Verification items for the finished model (mm, model axes). A direction names the side the tool comes from. Give positions to 0.01 mm unless a question says otherwise; leave off trailing zeros. Write each loop counter-clockwise with the first axis right and the second up, starting at its lowest first coordinate (ties: lowest second). Pieces come first, ordered by that corner, then holes. Notation, with made-up numbers: (-13.5, -5.75) - (35.5, -5.75) arc R13 cw to (35.5, -0.75) - close; hole circle Ø11 at (-3.5, 13). An arc over 180 degrees is marked (long way). Answer as a JSON object with one key per item and string values. Group by question number.
Item 1: Go/stop test with flat-tipped pins: pin 1 (7 mm diameter, centred on y = 0, z = 12.7, fed in from +X) (3 decimals); pin 2 (2 mm diameter, centred on x = -1.5, y = -6, fed in from +Z) (3 decimals); pin 3 (3 mm diameter, centred on x = 1.524, y = 0, fed in from -Z). Record where each tip stops, or that it passes through.
Item 2: Sectioned sample at B-B, the plane y = 12.7. Record the boundary of the cut face in (x, z) (3 decimals).
Item 3: Tool access check on faces 1 (the face through (-6.35, -0.3, 9.7)), 2 (the face through (-3.175, 0, 17)). Record the directions out of +Z, -Z, +X, -X, +Y, -Y that give a thin tool (end or side, any length) a straight path to the whole face; none if there is none.
Item 4: Sectioned sample at D-D, the plane x = 3.75. Record the boundary of the cut face in (y, z) (3 decimals).
Item 5: Scan lines: line 1 along X through (y, z) = (-12.7, 0.7); line 2 along Z through (x, y) = (-5.25, -12.7); line 3 along Y through (x, z) = (-3.25, 12.25). Record each from-to range of solid material in increasing order. Write a range as [from, to].
Item 6: Draft check along Y on faces 3 (the face through (-4, 19.05, 9)), 4 (the face through (5, 0, 3.175)), 5 (the face through (-4.74, 15.244, 13.501)). Enter one of: +Y half, -Y half, draft (parallel to the pull), parting line (faces both ways), or undercut.
Item 7: Sectioned sample at A-A, the plane z = 12.7. Record the boundary of the cut face in (x, y) (3 decimals), and give its area (3 significant figures).
Item 8: Sectioned sample at C-C, the plane z = 2.5. Record the boundary of the cut face in (x, y).
```python
from build123d import *

# Parameters (mm, degrees)
SKETCH1_W           = 19.05
SKETCH1_H           = 38.1
SKETCH1_R           = 2.667
BOSS_EXTRUDE1_DEPTH = 3.175
SKETCH2_W           = 3.175
SKETCH2_H           = 38.1
BOSS_EXTRUDE2_DEPTH = 22.225
SKETCH4_R           = 2.667
CUT_EXTRUDE1_DEPTH  = 36.497579143


with BuildPart() as part:
    # Sketch1 → Boss-Extrude1 (new body)
    with BuildSketch(Plane.XY):
        with Locations((3.175, 0)):
            Rectangle(SKETCH1_W, SKETCH1_H)
        with Locations(Location((1.524, -12.7, 0), (0, 0, 180))):
            Circle(SKETCH1_R, mode=Mode.SUBTRACT)
        with Locations(Location((1.524, 0, 0), (0, 0, 180))):
            Circle(SKETCH1_R, mode=Mode.SUBTRACT)
        with Locations(Location((1.524, 12.7, 0), (0, 0, 180))):
            Circle(SKETCH1_R, mode=Mode.SUBTRACT)
    extrude(amount=BOSS_EXTRUDE1_DEPTH)

    # Sketch2 → Boss-Extrude2 (add)
    with BuildSketch(Plane.XY.offset(3.175)):
        with Locations((-4.7625, 0)):
            Rectangle(SKETCH2_W, SKETCH2_H)
    extrude(amount=BOSS_EXTRUDE2_DEPTH)

    # Sketch4 → Cut-Extrude1 (cut, through all)
    with BuildSketch(Plane(origin=(-3.175, 0, 0), x_dir=(0, 0, -1), z_dir=(1, 0, 0))):
        with Locations(Location((-12.7, 0, 0), (0, 0, 90))):
            Circle(SKETCH4_R)
        with Locations(Location((-12.7, 12.7, 0), (0, 0, 90))):
            Circle(SKETCH4_R)
        with Locations(Location((-12.7, -12.7, 0), (0, 0, 90))):
            Circle(SKETCH4_R)
    extrude(amount=-CUT_EXTRUDE1_DEPTH, mode=Mode.SUBTRACT)


solid = part.part
```
Geometry check:
{
 "1": {"pin 1": "x = -3.175", "pin 2": "z = 3.175", "pin 3": "through"},
 "2": {"outline": "(-6.35, 0) - (-1.143, 0) - (-1.143, 3.175) - (-3.175, 3.175) - (-3.175, 10.033) - (-6.35, 10.033) - close; (-6.35, 15.367) - (-3.175, 15.367) - (-3.175, 25.4) - (-6.35, 25.4) - close; (4.191, 0) - (12.7, 0) - (12.7, 3.175) - (4.191, 3.175) - close"},
 "3": {"face 1": "+Z, -Z, -X, +Y, -Y", "face 2": "+Z, +X, +Y, -Y"},
 "4": {"outline": "(-19.05, 0) - (-14.169, 0) - (-14.169, 3.175) - (-19.05, 3.175) - close; (-11.231, 0) - (-1.469, 0) - (-1.469, 3.175) - (-11.231, 3.175) - close; (1.469, 0) - (11.231, 0) - (11.231, 3.175) - (1.469, 3.175) - close; (14.169, 0) - (19.05, 0) - (19.05, 3.175) - (14.169, 3.175) - close"},
 "5": {"line 1": "[-6.35, -1.14], [4.19, 12.7]", "line 2": "[0, 10.03], [15.37, 25.4]", "line 3": "[-19.05, -15.33], [-10.07, -2.63], [2.63, 10.07], [15.33, 19.05]"},
 "6": {"face 3": "+Y half", "face 4": "draft", "face 5": "undercut"},
 "7": {"outline": "(-6.35, -19.05) - (-3.175, -19.05) - (-3.175, -15.367) - (-6.35, -15.367) - close; (-6.35, -10.033) - (-3.175, -10.033) - (-3.175, -2.667) - (-6.35, -2.667) - close; (-6.35, 2.667) - (-3.175, 2.667) - (-3.175, 10.033) - (-6.35, 10.033) - close; (-6.35, 15.367) - (-3.175, 15.367) - (-3.175, 19.05) - (-6.35, 19.05) - close", "area": "70.2 mm^2"},
 "8": {"outline": "(-6.35, -19.05) - (12.7, -19.05) - (12.7, 19.05) - (-6.35, 19.05) - close; hole circle Ø5.33 at (1.52, -12.7); hole circle Ø5.33 at (1.52, 0); hole circle Ø5.33 at (1.52, 12.7)"}
}
